Can you work these out from the model? Positions are in its coordinate system, mm. A direction names the side the tool comes from. Round coordinates to 2 decimals unless told otherwise and drop trailing zeros. Loops run counter-clockwise (first coordinate to the right, second up) from the corner with the lowest first, then second, coordinate; pieces in that order, holes last. Notation, with made-up numbers: M 3.25,69 L 41.25,69 A27 cw 41.25,88 Z; hole C 23,65.25 d1. An arc over 180 degrees is marked long. Return JSON: item names as keys, results as strings.
```python
from build123d import *

# Parameters (mm, degrees)
SKETCH_1_R               = 7
EXTRUDE_1_DEPTH          = 2
SKETCH_2_R               = 6
EXTRUDE_2_DEPTH          = 35.5
CUT_EXTRUDE_1_DEPTH      = 39.784661917
CUT_EXTRUDE_1_DEPTH_BACK = 1.5
SKETCH_4_R               = 2
EXTRUDE_3_DEPTH          = 5
CUT_EXTRUDE_2_DEPTH      = 44.637713047
CUT_EXTRUDE_2_DEPTH_BACK = 44.637713047
CUT_EXTRUDE_6_OUTLINE_W  = 1.5
CUT_EXTRUDE_6_OUTLINE_H  = 7.50002714
PATTERN_LINEAR_2_COUNT   = 6
PATTERN_LINEAR_2_PITCH   = 4
CUT_EXTRUDE_7_DEPTH      = 1.5
FILLET_2_R               = 1.5
FILLET_3_R               = 1.5


# Read off the part's stored shape, not the designer's step: 切除-拉伸6
with BuildPart() as part:
    # 草图1 → 凸台-拉伸1 (new body)
    with BuildSketch(Plane(origin=(0, 0, 0), x_dir=(1, 0, 0), z_dir=(0, 1, 0))):
        with Locations(Location((0, 0, 0), (0, 0, 270))):
            Circle(SKETCH_1_R)
    extrude(amount=EXTRUDE_1_DEPTH)

    # 草图2 → 凸台-拉伸2 (add)
    with BuildSketch(Plane(origin=(0, 2, 0), x_dir=(1, 0, 0), z_dir=(0, 1, 0))):
        with Locations(Location((0, 0, 0), (0, 0, 270))):
            Circle(SKETCH_2_R)
    extrude(amount=EXTRUDE_2_DEPTH)

    # 草图3 → 切除-拉伸1 (cut, two sides: drawn at the far end of the back side and taken through both)
    with BuildSketch(Plane(origin=(0, 37.5, 0), x_dir=(1, 0, 0), z_dir=(0, 1, 0)).offset(-CUT_EXTRUDE_1_DEPTH_BACK)):
        with BuildLine():
            Line((0.0612495, -3.49946403), (-3.0612495, -1.696688392))
            ThreePointArc((-3.0612495, -1.696688392), (-1.75, -3.031088913), (0.0612495, -3.49946403))
        make_face()
        with BuildLine():
            ThreePointArc((0.0612495, -3.49946403), (-1.75, -3.031088913), (-3.0612495, -1.696688392))
            Line((-3.0612495, -1.696688392), (-6, 0))
            ThreePointArc((-6, 0), (-3, -5.196152423), (3, -5.196152423))
            Line((3, -5.196152423), (0.0612495, -3.49946403))
        make_face()
        with BuildLine():
            Line((-3, 5.196152423), (-0.0612495, 3.49946403))
            ThreePointArc((-0.0612495, 3.49946403), (1.75, 3.031088913), (3.0612495, 1.696688392))
            Line((3.0612495, 1.696688392), (6, 0))
            ThreePointArc((6, 0), (3, 5.196152423), (-3, 5.196152423))
        make_face()
        with BuildLine():
            ThreePointArc((3.0612495, 1.696688392), (1.75, 3.031088913), (-0.0612495, 3.49946403))
            Line((-0.0612495, 3.49946403), (3.0612495, 1.696688392))
        make_face()
    extrude(amount=CUT_EXTRUDE_1_DEPTH + CUT_EXTRUDE_1_DEPTH_BACK, mode=Mode.SUBTRACT)

    # 草图4 → 凸台-拉伸3 (add)
    with BuildSketch(Plane(origin=(0, 37.5, 0), x_dir=(1, 0, 0), z_dir=(0, 1, 0))):
        with Locations(Location((3.031088913, -1.75, 0), (0, 0, 270))):
            Circle(SKETCH_4_R)
        with Locations(Location((-3.031088913, 1.75, 0), (0, 0, 270))):
            Circle(SKETCH_4_R)
    extrude(amount=EXTRUDE_3_DEPTH)

    # 草图5 → 切除-拉伸2 (cut, two sides: drawn at the far end of the back side and taken through both)
    with BuildSketch(Plane(origin=(0, 0, 0), x_dir=(1, 0, 0), z_dir=(0, 1, 0)).offset(-CUT_EXTRUDE_2_DEPTH_BACK)):
        Polygon((-1.35, 49.247498963), (-1.35, 6.868587919), (-1.35, 4.2), (0, 4.2), (0, 2.7), (-0.75, 2.7), (-0.75, -2.5), (0.75, -2.5), (0.75, 1.5), (1.353400632, 1.5), (1.353400632, 6.867918661), (1.353400632, 49.246829705), (1.374383416, 134.004649195), (-1.329017216, 134.005318453), align=None)
    extrude(amount=CUT_EXTRUDE_2_DEPTH + CUT_EXTRUDE_2_DEPTH_BACK, mode=Mode.SUBTRACT)

    # 切除-拉伸6 outline → 切除-拉伸6 (revolve, cut)
    with BuildSketch(Plane.XZ.offset(-27.6)):
        with Locations((0.75, 2.25001357)):
            Rectangle(CUT_EXTRUDE_6_OUTLINE_W, CUT_EXTRUDE_6_OUTLINE_H)
    cut_extrude_6 = revolve(axis=Axis((0, 27.6, 0), (0, 0, 1)), mode=Mode.SUBTRACT)

    # 阵列(线性)2: 切除-拉伸6 ×6
    with Locations(*[(0, -i * PATTERN_LINEAR_2_PITCH, 0) for i in range(1, PATTERN_LINEAR_2_COUNT)]):
        add(cut_extrude_6, mode=Mode.SUBTRACT)

    # 草图15 → 切除-拉伸7 (cut, symmetric)
    with BuildSketch(Plane(origin=(0, 3.6, 0), x_dir=(1, 0, 0), z_dir=(0, 1, 0))):
        with BuildLine():
            Line((0, -6), (0, -4.5))
            ThreePointArc((0, -4.5), (-1.803051209, -4.122985125), (-3.303979251, -3.055113928))
            Line((-3.303979251, -3.055113928), (-4.36524821, -4.116382886))
            ThreePointArc((-4.36524821, -4.116382886), (-2.377151939, -5.509006141), (0, -6))
        make_face()
    extrude(amount=CUT_EXTRUDE_7_DEPTH, both=True, mode=Mode.SUBTRACT)

    # 圆角2
    fillet_2_edges = [part.edges().sort_by_distance(p)[0] for p in [
        (0, 5.1, 5.25),
        (0, 2.1, 5.25),
    ]]
    fillet(fillet_2_edges, radius=FILLET_2_R - 0.0001)  # a hair under: the kernel refuses the full size

    # 圆角3
    fillet_3_edges = [part.edges().sort_by_distance(p)[0] for p in [
        (-3.83461373, 2.1, 3.585748407),
        (-3.83461373, 5.1, 3.585748407),
    ]]
    fillet(fillet_3_edges, radius=FILLET_3_R - 0.0001)  # a hair under: the kernel refuses the full size


solid = part.part
```
Q1. Suppose I cut it at A-A, the plane y = 15.6. Please give me the cut outline in (x, z), plus the area to 3 significant figures.
Results:
{"outline": "M -1.5,-1.5 L -1.5,5.81 A6 ccw -1.35,-5.85 L -1.35,-4.2 L 0,-4.2 L 0,-2.7 L -0.75,-2.7 L -0.75,-1.5 Z; M 1.35,-5.85 A6 ccw 1.5,5.81 L 1.5,-1.5 L 1.35,-1.5 Z", "area": "81.5 mm2"}
Q2. Thinking about a two-plate mould opening in Y: for faces 4 (the flat face through (4, 36, -3)), 5 (the cylindrical face through (-0.195, 29.087, 3.136)), 6 (the cylindrical face through (-0.195, 25.087, 3.136)), 7 (the flat face through (0.75, 33, 1)), which applies, pulls with the +Y half, pulls with the -Y half, needs draft (parallel to the pull), parting line crosses it, or undercut?
Results:
{"face 4": "pulls with the +Y half", "face 5": "undercut", "face 6": "undercut", "face 7": "needs draft"}
Q3. If I drill on line 1 along X through (y, z) = (35, -4.25); line 2 along Z through (x, y) = (-3, 12.5); line 3 along X through (y, z) = (23.5, -3), over which ranges is the centre line in solid material (lowest first)?
Results:
{"line 1": "x = -4.24 to -1.35, 1.35 to 4.24", "line 2": "z = -5.2 to 5.2", "line 3": "x = -5.2 to 0, 1.35 to 5.2"}
Q4. On a 3-axis mill with a long thin cutter (end or side, diameter ignored), from which of +Z, -Z, +X, -X, +Y, -Y can I reach the whole of each face in a straight line? I mean faces 1 (the flat face through (2, 2, 6)), 2 (the flat face through (0, 9.6, 2.5)), 3 (the flat face through (-1.35, 18, -5)). Say none if no direction works.
Results:
{"face 1": "+Y", "face 2": "+Y, -Y", "face 3": "-Z, +Y, -Y"}
Q5. I'm going to push flat-ended pins straight in: pin 1 Ø5 at (y, z) = (12.5, 4) entering from -X; pin 2 Ø1.5 at (x, y) = (0, 26) entering from -Z; pin 3 Ø0.7 at (y, z) = (21.5, 0) entering from -X. Where does each tip first touch, or does it pass through?
Results:
{"pin 1": "stops at x = -5.81", "pin 2": "stops at z = -4.2", "pin 3": "stops at x = -6"}
